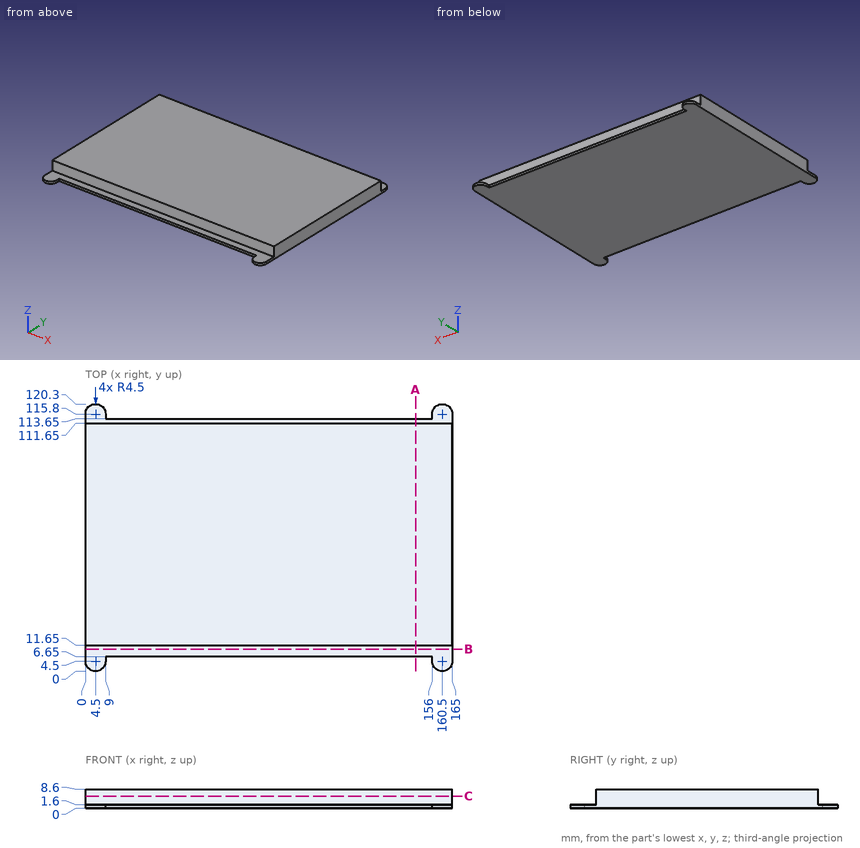
Here's the drawing with two shaded views (mm, measured from the low corner). I have some questions. Give positions to 0.01 mm unless a question says otherwise; leave off trailing zeros. Write each loop counter-clockwise with the first axis right and the second up, starting at its lowest first coordinate (ties: lowest second). Pieces come first, ordered by that corner, then holes. Notation, with made-up numbers: (70.25, 40.25) -> (84.25, 40.25) arc R11 cw to (84.25, 45.25) -> close; hole circle Ø5 at (52, 7.5). An arc over 180 degrees is marked (long way). One line per item, written item: value.
Q1. Imagine slicing it at C-C on z = 5.5. Please give me the cut outline in (x, y), and give its area (3 significant figures).
Results found:
outline: (0, 11.65) -> (165, 11.65) -> (165, 111.65) -> (0, 111.65) -> close
area: 16,500 mm^2
Q2. Please list where these lines run through material, in increasing order: line 1 (Y direction, x = 157, z = 6.75); line 2 (Z direction, x = 99, y = 8); line 3 (Y direction, x = 117.5, z = 1.25). Write a range as [from, to].
Results found:
line 1: y = [11.65, 111.65]
line 2: z = [0, 1.6]
line 3: y = [6.65, 113.65]
Q3. Imagine slicing it at B-B on y = 10. Please give me the cut outline in (x, z).
Results found:
outline: (0, 0) -> (165, 0) -> (165, 1.6) -> (0, 1.6) -> close
Q4. Imagine slicing it at A-A on x = 148.5. Please give me the cut outline in (y, z), and give its area (3 significant figures).
Results found:
outline: (6.65, 0) -> (113.65, 0) -> (113.65, 1.6) -> (111.65, 1.6) -> (111.65, 8.6) -> (11.65, 8.6) -> (11.65, 1.6) -> (6.65, 1.6) -> close
area: 871 mm^2
Q5. For P1, Ø5, axis at x = 58, z = 7.5, coming from the -Y side; P2, Ø5, axis at x = 43, y = 57.5, coming from the -Z side; P3, Ø7, axis at x = 112.5, y = 118, coming from the +Z side; P4, Ø3, axis at x = 80.5, z = 3.5, coming from the +Y side, each with a flat end and sliding along its axis, tell me the tip position at first contact or that it passes through.
Results found:
P1: stops at y = 11.65
P2: stops at z = 0
P3: passes through
P4: stops at y = 111.65
